Design review of the part built by this model. Coordinates are the model's own, in mm. A direction names the side the tool comes from. Give positions to 0.01 mm unless a question says otherwise; leave off trailing zeros. Write each loop counter-clockwise with the first axis right and the second up, starting at its lowest first coordinate (ties: lowest second). Pieces come first, ordered by that corner, then holes. Notation, with made-up numbers: (53.25, 35.5) -> (106.25, 35.5) arc R25 cw to (106.25, 62.5) -> close; hole circle Ø11 at (-4, 44). An arc over 180 degrees is marked (long way). Use CSV: the item, a comma, the result in double quotes.
```python
from build123d import *

# Parameters (mm, degrees)
F0_W     = 25.4
F0_H     = 609.6
F1_DEPTH = 19.05
F2_W     = 19.05
F2_H     = 25.4
F3_DEPTH = 19.05
F4_W     = 19.05
F4_H     = 25.4
F5_DEPTH = 19.05


with BuildPart() as f1:
    # F0 (on Front) → F1 (new body)
    with BuildSketch(Plane.XZ):
        with Locations((-12.7, -304.8)):
            Rectangle(F0_W, F0_H)
    extrude(amount=F1_DEPTH)

    # F2 (on face) → F3 (join)
    with BuildSketch(Plane(origin=(-25.4, 0, 0), x_dir=(0, -1, 0), z_dir=(-1, 0, 0))):
        with Locations((9.525, -50.8)):
            Rectangle(F2_W, F2_H)
    extrude(amount=F3_DEPTH)

    # F4 (on face) → F5 (join)
    with BuildSketch(Plane.YZ):
        with Locations((-9.525, -533.4)):
            Rectangle(F4_W, F4_H)
    extrude(amount=F5_DEPTH)


solid = f1.part
```
(1) Clearance check with flat-ended pins moving along their axes: pin 1 (9.5 mm diameter, centred on x = 6, y = -7, fed in from +Z); pin 2 (1 mm diameter, centred on y = -5, z = -386.5, fed in from +X); pin 3 (5.5 mm diameter, centred on x = -38, y = -5.5, fed in from +Z). State where each tip first meets the part, or that it passes through.
Established:
pin 1,"stops at z = -520.7"
pin 2,"stops at x = 0"
pin 3,"stops at z = -38.1"
(2) Tool access review of faces 1 (the face through (-44.45, -9, -51)), 2 (the face through (0, -9, -578)), 3 (the face through (9, -10, -520.7)), 4 (the face through (-35, -9, -38.1)), 5 (the face through (-25.4, -9, -340)): name each direction out of +Z, -Z, +X, -X, +Y, -Y from which nothing blocks a thin tool from reaching the whole face with its end or side.
Established:
face 1,"+Z, -Z, -X, +Y, -Y"
face 2,"-Z, +X, +Y, -Y"
face 3,"+Z, +X, +Y, -Y"
face 4,"+Z, -X, +Y, -Y"
face 5,"-Z, -X, +Y, -Y"
(3) Take a section at B-B (x = 8.5). Write out the cut boundary in (y, z), then the cut area to 3 significant figures.
Established:
outline,"(-19.05, -546.1) -> (0, -546.1) -> (0, -520.7) -> (-19.05, -520.7) -> close"
area,"484 mm2"
(4) Take a section at A-A (y = -4). Write out the cut boundary in (x, z), then the cut area to 3 significant figures.
Established:
outline,"(-44.45, -63.5) -> (-25.4, -63.5) -> (-25.4, -609.6) -> (0, -609.6) -> (0, -546.1) -> (19.05, -546.1) -> (19.05, -520.7) -> (0, -520.7) -> (0, 0) -> (-25.4, 0) -> (-25.4, -38.1) -> (-44.45, -38.1) -> close"
area,"16,500 mm2"
(5) Take a section at C-C (z = -116). Write out the cut boundary in (x, y), then the cut area to 3 significant figures.
Established:
outline,"(-25.4, -19.05) -> (0, -19.05) -> (0, 0) -> (-25.4, 0) -> close"
area,"484 mm2"
(6) For line 1 along X through (y, z) = (-4.75, -452.5); line 2 along X through (y, z) = (-8.25, -527); line 3 along Z through (x, y) = (-25.5, -12.5), list the stretches that pass through material, from the lowest coordinate up. Write a range as [from, to].
Established:
line 1,"x = [-25.4, 0]"
line 2,"x = [-25.4, 19.05]"
line 3,"z = [-63.5, -38.1]"
